```python
from build123d import *

# Parameters (mm, degrees)
F0_W     = 70
F0_H     = 70
F1_DEPTH = 5
F3_DEPTH = 3
F5_DEPTH = 25


with BuildPart() as f1:
    # F0 (on Top) → F1 (new body)
    with BuildSketch(Plane.XY):
        Rectangle(F0_W, F0_H)
    extrude(amount=F1_DEPTH)

    # F2 (on face) → F3 (cut)
    with BuildSketch(Plane.XY.offset(5)):
        Polygon((-29, -24.727326), (-29, -29), (-24.344364, -29), (-24.118565, -28.495094), (-26.996544, -24.520101), align=None)
        Polygon((-24.344364, -29), (-29, -29), (-29, -24.727326), (-31.877979, -25.025007), (-33.881435, -29.504906), (-31.003456, -33.479899), (-26.122021, -32.974993), align=None)
        Polygon((24.118565, -28.495094), (24.344364, -29), (29, -29), (29, -24.727326), (26.996544, -24.520101), align=None)
        Polygon((29, -29), (24.344364, -29), (26.122021, -32.974993), (31.003456, -33.479899), (33.881435, -29.504906), (31.877979, -25.025007), (29, -24.727326), align=None)
        Polygon((-31.003456, 24.520101), (-29, 24.727326), (-29, 29), (-24.344364, 29), (-24.118565, 29.504906), (-26.996544, 33.479899), (-31.877979, 32.974993), (-33.881435, 28.495094), align=None)
        Polygon((-29, 29), (-29, 24.727326), (-26.122021, 25.025007), (-24.344364, 29), align=None)
        Polygon((26.996544, 24.520101), (29, 24.727326), (29, 29), (24.344364, 29), (24.118565, 28.495094), align=None)
        Polygon((29, 29), (29, 24.727326), (31.877979, 25.025007), (33.881435, 29.504906), (31.003456, 33.479899), (26.122021, 32.974993), (24.344364, 29), align=None)
    extrude(amount=-F3_DEPTH, mode=Mode.SUBTRACT)

    # F4 (on face) → F5 (cut)
    with BuildSketch(Plane.XY.offset(5)):
        with BuildLine():
            Line((-29, -27.125), (-29, -29))
            Line((-29, -29), (-27.125, -29))
            ThreePointArc((-27.125, -29), (-27.674175, -27.674175), (-29, -27.125))
        make_face()
        with BuildLine():
            Line((-27.125, -29), (-29, -29))
            Line((-29, -29), (-29, -27.125))
            ThreePointArc((-29, -27.125), (-30.325825, -30.325825), (-27.125, -29))
        make_face()
        with BuildLine():
            ThreePointArc((29, -27.125), (27.674175, -27.674175), (27.125, -29))
            Line((27.125, -29), (29, -29))
            Line((29, -29), (29, -27.125))
        make_face()
        with BuildLine():
            Line((29, -29), (27.125, -29))
            ThreePointArc((27.125, -29), (29, -30.875), (30.875, -29))
            ThreePointArc((30.875, -29), (30.325825, -27.674175), (29, -27.125))
            Line((29, -27.125), (29, -29))
        make_face()
        with BuildLine():
            ThreePointArc((-27.125, 29), (-30.325825, 30.325825), (-29, 27.125))
            Line((-29, 27.125), (-29, 29))
            Line((-29, 29), (-27.125, 29))
        make_face()
        with BuildLine():
            Line((-29, 29), (-29, 27.125))
            ThreePointArc((-29, 27.125), (-27.674175, 27.674175), (-27.125, 29))
            Line((-27.125, 29), (-29, 29))
        make_face()
        with BuildLine():
            Line((29, 29), (27.125, 29))
            ThreePointArc((27.125, 29), (27.674175, 27.674175), (29, 27.125))
            Line((29, 27.125), (29, 29))
        make_face()
        with BuildLine():
            ThreePointArc((30.875, 29), (29, 30.875), (27.125, 29))
            Line((27.125, 29), (29, 29))
            Line((29, 29), (29, 27.125))
            ThreePointArc((29, 27.125), (30.325825, 27.674175), (30.875, 29))
        make_face()
    extrude(amount=-F5_DEPTH, mode=Mode.SUBTRACT)


solid = f1.part
```
CAD build for the part. Positions are in the model's coordinates, mm. A direction names the side the tool comes from. Give positions to 0.01 mm unless a question says otherwise; leave off trailing zeros. Write each loop counter-clockwise with the first axis right and the second up, starting at its lowest first coordinate (ties: lowest second). Pieces come first, ordered by that corner, then holes. Notation, with made-up numbers: M 58,4 L 102,4 A25 ccw 102,26 Z; hole C -26,27.5 d2. An arc over 180 degrees is marked long. Return JSON: item names as keys, results as strings. Group by question number.
(1) Drill centre lines: L1, parallel to Y at x = -29, z = 0.6 (3 decimals); L2, parallel to X at y = 32, z = 4.3. Where is each one in solid material? Low to high. Write a range as [from, to].
(2) Band-saw the part on B-B (z = 3.1). State how many separate pieces and enclosed holes the cut face has, and give its area (3 significant figures).
(3) Band-saw the part on A-A (x = -30). Give the cut face in (y, z), and give its area (3 significant figures).
(4) 3-axis set-ups, long thin cutter, end or side, ignore diameter. For faces 5 (the face through (-25.537, 31.465, 3.521)), 6 (the face through (-35, 0, 2)): which of +Z, -Z, +X, -X, +Y, -Y reach the whole face in a straight line?
(5) Flat gauge pins, fed straight in: pin 1 Ø8 at (x, y) = (-9, 22) entering from -Z; pin 2 Ø2.5 at (x, y) = (-29.5, -27.5) entering from +Z. Where does each tip first touch, or does it go through?
(6) Mould opens along Y. For faces 1 (the face through (35, 0, 2)), 2 (the face through (0, -35, 2)), 3 (the face through (32.866, 27.234, 3.521)), 4 (the face through (28.6, 33.23, 3.52)) say: pulls with the +Y half, pulls with the -Y half, needs draft (parallel to the pull), parting line crosses it, or undercut.
Entries:
{
 "1": {"L1": "y = [-35, -30.875], [-27.125, 27.125], [30.875, 35]", "L2": "x = [-35, -32.31], [-25.93, 25.69], [32.07, 35]"},
 "2": {"separate pieces": "1", "enclosed holes": "4", "area": "4,650 mm^2"},
 "3": {"outline": "M -35,0 L -30.59,0 L -30.59,2 L -33.38,2 L -33.38,5 L -35,5 Z; M -27.41,0 L 27.41,0 L 27.41,2 L 24.62,2 L 24.62,5 L -24.83,5 L -24.83,2 L -27.41,2 Z; M 30.59,0 L 35,0 L 35,5 L 33.17,5 L 33.17,2 L 30.59,2 Z", "area": "286 mm^2"},
 "4": {"face 5": "+Z", "face 6": "+Z, -Z, -X, +Y, -Y"},
 "5": {"pin 1": "stops at z = 0", "pin 2": "stops at z = 2"},
 "6": {"face 1": "needs draft", "face 2": "pulls with the -Y half", "face 3": "undercut", "face 4": "undercut"}
}
